Read the model definition and answer for the solid it produces. Units are mm, in the model's axes. Face numbers are marked on the shaded views. A direction names the side the tool comes from. Coordinates: 2 decimals unless noted, no trailing zeros. Order: outer loops, then holes, each group sorted by start corner. A loop starts at its lowest first (then second) coordinate and runs counter-clockwise, first axis right, second up. Notation, with made-up numbers: M 13.5,75.5 L 43.5,75.5 A12 ccw 43.5,82.5 Z; hole C 28,13.25 d3. An arc over 180 degrees is marked long. Write each question's results on one line, items separated by ' | '.
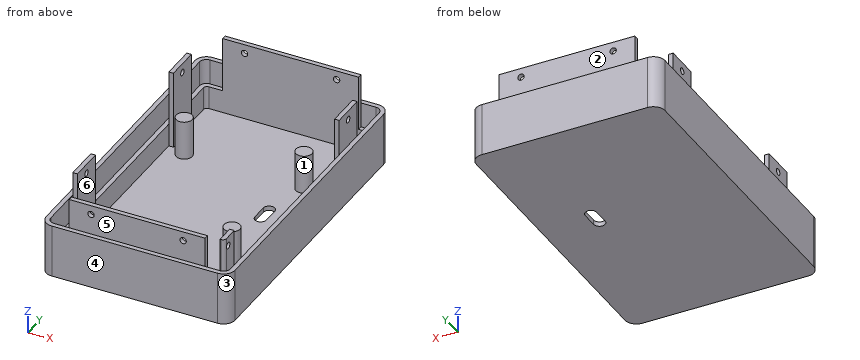
```python
from build123d import *

# Parameters (mm, degrees)
F1_DEPTH  = 23
F2_T      = -2
F3_R      = 3.5
F4_DEPTH  = 17
F5_DEPTH  = 2
F6_DEPTH  = 10
F7_W      = 59
F7_H      = 2
F7_W_2    = 2
F7_H_2    = 15
F8_DEPTH  = 34
F9_R      = 1.4
F10_DEPTH = 132.001
F11_R     = 1.4
F12_DEPTH = 78.001


with BuildPart() as f1:
    # F0 (on Top) → F1 (new body)
    with BuildSketch(Plane.XY):
        with BuildLine():
            Line((-36, -67), (36, -67))
            ThreePointArc((36, -67), (39.5355339059, -65.5355339059), (41, -62))
            Line((41, -62), (41, 62))
            ThreePointArc((41, 62), (39.5355339059, 65.5355339059), (36, 67))
            Line((36, 67), (-36, 67))
            ThreePointArc((-36, 67), (-39.5355339059, 65.5355339059), (-41, 62))
            Line((-41, 62), (-41, -62))
            ThreePointArc((-41, -62), (-39.5355339059, -65.5355339059), (-36, -67))
        make_face()
    extrude(amount=F1_DEPTH)

    # F2
    f2_openings = [f1.faces().sort_by_distance(p)[0] for p in [
        (0, 0, 23),
    ]]
    offset(amount=F2_T, openings=f2_openings)

    # F3 (on face) → F4 (join)
    with BuildSketch(Plane.XY.offset(2)):
        with Locations((-29, 30)):
            Circle(F3_R)
        with Locations((23, 30)):
            Circle(F3_R)
        with Locations((23, -30)):
            Circle(F3_R)
    extrude(amount=F4_DEPTH)

    # F3 (on face) → F5 (cut)
    with BuildSketch(Plane.XY.offset(2)):
        with BuildLine():
            ThreePointArc((15.5, 3.5), (18, 1), (20.5, 3.5))
            Line((20.5, 3.5), (20.5, 10.5))
            ThreePointArc((20.5, 10.5), (18, 13), (15.5, 10.5))
            Line((15.5, 10.5), (15.5, 3.5))
        make_face()
    extrude(amount=-F5_DEPTH, mode=Mode.SUBTRACT)

    # F3 (on face) → F6 (join)
    with BuildSketch(Plane.XY.offset(2)):
        with BuildLine():
            Line((-36, -65), (36, -65))
            ThreePointArc((36, -65), (38.1213203436, -64.1213203436), (39, -62))
            Line((39, -62), (39, 62))
            ThreePointArc((39, 62), (38.1213203436, 64.1213203436), (36, 65))
            Line((36, 65), (-36, 65))
            ThreePointArc((-36, 65), (-38.1213203436, 64.1213203436), (-39, 62))
            Line((-39, 62), (-39, -62))
            ThreePointArc((-39, -62), (-38.1213203436, -64.1213203436), (-36, -65))
        make_face()
        with BuildLine():
            ThreePointArc((37, -61.5), (36.5606601718, -62.5606601718), (35.5, -63))
            Line((35.5, -63), (-35.5, -63))
            ThreePointArc((-35.5, -63), (-36.5606601718, -62.5606601718), (-37, -61.5))
            Line((-37, -61.5), (-37, 61.5))
            ThreePointArc((-37, 61.5), (-36.5606601718, 62.5606601718), (-35.5, 63))
            Line((-35.5, 63), (35.5, 63))
            ThreePointArc((35.5, 63), (36.5606601718, 62.5606601718), (37, 61.5))
            Line((37, 61.5), (37, -61.5))
        make_face(mode=Mode.SUBTRACT)
    extrude(amount=F6_DEPTH)

    # F7 (on face) → F8 (join)
    with BuildSketch(Plane.XY.offset(2)):
        with Locations((0, 64)):
            Rectangle(F7_W, F7_H)
        with Locations((0, -64)):
            Rectangle(F7_W, F7_H)
        with Locations((-36, 40)):
            Rectangle(F7_W_2, F7_H_2)
        with Locations((-36, -40)):
            Rectangle(F7_W_2, F7_H_2)
        with Locations((36, 40)):
            Rectangle(F7_W_2, F7_H_2)
        with BuildLine():
            Line((37, -61.5), (37, -55))
            Line((37, -55), (35, -55))
            Line((35, -55), (35, -63))
            Line((35, -63), (35.5, -63))
            ThreePointArc((35.5, -63), (36.5606601718, -62.5606601718), (37, -61.5))
        make_face()
    extrude(amount=F8_DEPTH)

    # F9 (on face) → F10 (cut, through all)
    with BuildSketch(Plane.XZ.offset(65)):
        with Locations((-20, 32)):
            Circle(F9_R)
        with Locations((20, 32)):
            Circle(F9_R)
    extrude(amount=-F10_DEPTH, mode=Mode.SUBTRACT)

    # F11 (on face) → F12 (cut, through all)
    with BuildSketch(Plane.YZ.offset(37)):
        with Locations((40, 32)):
            Circle(F11_R)
        with Locations((-40, 32)):
            Circle(F11_R)
        with Locations((-60, 32)):
            Circle(F11_R)
    extrude(amount=-F12_DEPTH, mode=Mode.SUBTRACT)


solid = f1.part
```
(1) Straight lines are drawn through the part: line 1 (X direction, y = 40, z = 15.5); line 2 (Y direction, x = -7, z = 22.5); line 3 (X direction, y = -35.5, z = 16). For each, find the intervals that lie inside material, in ascending order.
Conclusion:
line 1: -41 to -39, -37 to -35, 35 to 37, 39 to 41 | line 2: -67 to -63, 63 to 67 | line 3: -41 to -39, -37 to -35, 39 to 41
(2) The part is cut by section D-D, the plane x = -2. Write down the section's boundary in (y, z).
Conclusion:
outline: M -67,0 L 67,0 L 67,23 L 65,23 L 65,36 L 63,36 L 63,2 L -63,2 L -63,36 L -65,36 L -65,23 L -67,23 Z
(3) The mould has two halves that part along X. Classify the marked faces 1, 2 and 3: pulls with the +X half, pulls with the -X half, needs draft (parallel to the pull), parting line crosses it, or undercut.
Conclusion:
face 1: undercut | face 2: needs draft | face 3: pulls with the +X half
(4) The part is cut by section B-B, the plane x = -20. Write down the section's boundary in (y, z), then the cut area to 3 significant figures.
Conclusion:
outline: M -67,0 L 67,0 L 67,23 L 65,23 L 65,30.6 L 63,30.6 L 63,2 L -63,2 L -63,30.6 L -65,30.6 L -65,23 L -67,23 Z; M -65,33.4 L -63,33.4 L -63,36 L -65,36 Z; M 63,33.4 L 65,33.4 L 65,36 L 63,36 Z | area: 477 mm²
(5) The part is cut by section A-A, the plane z = 9. Count the separate pieces of the cut face and the enclosed holes in it, then the cut area to 3 significant figures.
Conclusion:
separate pieces: 4 | enclosed holes: 1 | area: 1,870 mm²
(6) For the marked faces 4, 5 and 6, determine the directions among +Z, -Z, +X, -X, +Y, -Y from which every point of the face is accessible in a straight line to the end or side of a thin tool.
Conclusion:
face 4: +Z, -Z, +X, -X, -Y | face 5: +Z, +X, -X, -Y | face 6: +Z
(7) The part is cut by section C-C, the plane y = -22.5. Write down the section's boundary in (x, z), then the cut area to 3 significant figures.
Conclusion:
outline: M -41,0 L 41,0 L 41,23 L 39,23 L 39,12 L 37,12 L 37,2 L -37,2 L -37,12 L -39,12 L -39,23 L -41,23 Z | area: 288 mm²
(8) Given pin 1 (1 mm diameter, centred on x = -6, y = 24.5, fed in from +Z); pin 2 (6 mm diameter, centred on x = 7, z = 30.5, fed in from +Y); pin 3 (1.6 mm diameter, centred on y = 63.5, z = 25, fed in from -X), each flat-ended and moving along its own axis, determine where each tip first touches the part or whether it passes through.
Conclusion:
pin 1: z = 2 | pin 2: y = 65 | pin 3: x = -29.5
